Source: CAD feature listing. Evaluate the final solid. Frame: model axes, mm. Round coordinates to 2 decimals unless told otherwise and drop trailing zeros. Loops run counter-clockwise (first coordinate to the right, second up) from the corner with the lowest first, then second, coordinate; pieces in that order, holes last. Notation, with made-up numbers: (84, -18.75) - (93, -18.75) arc R29 ccw to (93, 10.25) - close; hole circle Ø5 at (-13.75, 24). An arc over 180 degrees is marked (long way). One line per question, with ' | ' between items.
from build123d import *

# Parameters (mm, degrees)
SKETCH1_W                      = 101.6
SKETCH1_H                      = 76.2
BOSS_EXTRUDE1_DEPTH            = 8.89
TAP_DRILL_FOR_M6X1_0_TAP1_D    = 5
CBORE_FOR_M6_SHCS1_D           = 6.6
CBORE_FOR_M6_SHCS1_CBORE_D     = 9.4
CBORE_FOR_M6_SHCS1_CBORE_DEPTH = 6.3


with BuildPart() as part:
    # Sketch1 → Boss-Extrude1 (new body)
    with BuildSketch(Plane(origin=(0, 0, 0), x_dir=(1, 0, 0), z_dir=(0, 1, 0))):
        Rectangle(SKETCH1_W, SKETCH1_H)
    extrude(amount=BOSS_EXTRUDE1_DEPTH)

    # Tap Drill for M6x1.0 Tap1 (through all)
    with Locations(Plane(origin=(0, 8.89, 0), x_dir=(1, 0, 0), z_dir=(0, 1, 0))):
        with Locations((-25.4, 25.4), (25.4, 25.4), (25.4, -25.4), (-25.4, -25.4)):
            Hole(TAP_DRILL_FOR_M6X1_0_TAP1_D / 2)

    # CBORE for M6 SHCS1 (through all)
    with Locations(Plane(origin=(0, 8.89, 0), x_dir=(1, 0, 0), z_dir=(0, 1, 0))):
        with Locations((-25.4, 12.7), (-25.4, -12.7), (0, -12.7), (0, 12.7), (25.4, 12.7), (25.4, -12.7)):
            CounterBoreHole(CBORE_FOR_M6_SHCS1_D / 2, CBORE_FOR_M6_SHCS1_CBORE_D / 2, CBORE_FOR_M6_SHCS1_CBORE_DEPTH)


solid = part.part
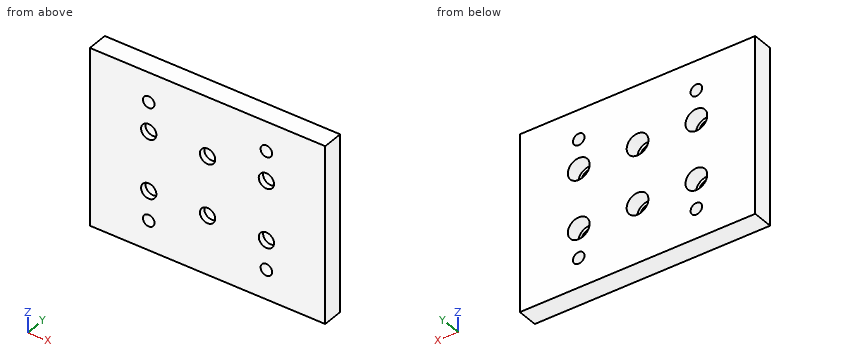
1. Section query C-C, the plane y = 1.5. Give the number of separate pieces and of enclosed holes in the cut face, plus the area to 3 significant figures.
Worked out:
separate pieces: 1 | enclosed holes: 10 | area: 7,460 mm2
2. Section query A-A, the plane z = -25.4. Return loops of the section in (x, y), plus the area to 3 significant figures.
Worked out:
outline: (-50.8, 0) - (-27.9, 0) - (-27.9, 8.89) - (-50.8, 8.89) - close; (-22.9, 0) - (22.9, 0) - (22.9, 8.89) - (-22.9, 8.89) - close; (27.9, 0) - (50.8, 0) - (50.8, 8.89) - (27.9, 8.89) - close | area: 814 mm2
3. Material intervals for probe 1 along X at (y, z) = (5.25, -25.5); probe 2 along Z at (x, y) = (0, 1.4); probe 3 along Z at (x, y) = (-25.4, 7), sorted ascending.
Worked out:
probe 1: x = -50.8 to -27.9, -22.9 to 22.9, 27.9 to 50.8 | probe 2: z = -38.1 to -16, -9.4 to 9.4, 16 to 38.1 | probe 3: z = -38.1 to -27.9, -22.9 to -17.4, -8 to 8, 17.4 to 22.9, 27.9 to 38.1
4. Section query B-B, the plane x = 0. Return loops of the section in (y, z), plus the area to 3 significant figures.
Worked out:
outline: (0, -38.1) - (8.89, -38.1) - (8.89, -17.4) - (2.59, -17.4) - (2.59, -16) - (0, -16) - close; (0, -9.4) - (2.59, -9.4) - (2.59, -8) - (8.89, -8) - (8.89, 8) - (2.59, 8) - (2.59, 9.4) - (0, 9.4) - close; (0, 16) - (2.59, 16) - (2.59, 17.4) - (8.89, 17.4) - (8.89, 38.1) - (0, 38.1) - close | area: 525 mm2
5. Contact query for a flat-ended pin moving along its axis: P1, Ø7.5, axis at x = -25.4, z = -12.7, coming from the +Y side. Output: stop coordinate, or through.
Worked out:
P1: stops at y = 2.59
6. Section query D-D, the plane x = -25.4. Return loops of the section in (y, z).
Worked out:
outline: (0, -38.1) - (8.89, -38.1) - (8.89, -27.9) - (0, -27.9) - close; (0, -22.9) - (8.89, -22.9) - (8.89, -17.4) - (2.59, -17.4) - (2.59, -16) - (0, -16) - close; (0, -9.4) - (2.59, -9.4) - (2.59, -8) - (8.89, -8) - (8.89, 8) - (2.59, 8) - (2.59, 9.4) - (0, 9.4) - close; (0, 16) - (2.59, 16) - (2.59, 17.4) - (8.89, 17.4) - (8.89, 22.9) - (0, 22.9) - close; (0, 27.9) - (8.89, 27.9) - (8.89, 38.1) - (0, 38.1) - close
